Model file for the job. Use its own axes, mm. A direction names the side the tool comes from. Round coordinates to 2 decimals unless told otherwise and drop trailing zeros. Loops run counter-clockwise (first coordinate to the right, second up) from the corner with the lowest first, then second, coordinate; pieces in that order, holes last. Notation, with made-up numbers: (-32, 85.25) - (-22, 85.25) arc R14 ccw to (-22, 93.25) - close; hole circle Ø4 at (-33, 77). An arc over 180 degrees is marked (long way). Answer as a JSON object with one key per item and string values.
from build123d import *

# Parameters (mm, degrees)
BOX039_W                 = 5
BOX039_H                 = 12
BOX039_DEPTH             = 7.5
CYLINDER041_R            = 1.75
CYLINDER041_DEPTH        = 32
PRISM_DEPTH              = 10
SKETCH009_R              = 1
SKETCH009_W              = 24
SKETCH009_H              = 13
PAD004_DEPTH             = 30
CYLINDER039_R            = 1.75
CYLINDER039_DEPTH        = 32
CYLINDER039_ROLL_ANGLE   = -90
CYLINDER040_R            = 1.75
CYLINDER040_DEPTH        = 32
CYLINDER040_ROLL_ANGLE   = -90
BOX026_W                 = 19
BOX026_H                 = 15
BOX026_DEPTH             = 56
CHAMFER005_SIZE          = 3
FILLET054_R              = 0.5
CLONE013_PLACEMENT_ANGLE = -90


with BuildPart() as cubo015:
    # Box039 → Box039 (new body)
    with BuildSketch(Plane(origin=(9, 97, 127), x_dir=(1, 0, 0), z_dir=(0, 0, 1))):
        with Locations((2.5, 6)):
            Rectangle(BOX039_W, BOX039_H)
    extrude(amount=BOX039_DEPTH)


with BuildPart() as cilindro016:
    # Cylinder041 → Cylinder041 (new body)
    with BuildSketch(Plane(origin=(-5, 104, 125.85), x_dir=(0, -1, 0), z_dir=(1, 0, 0))):
        Circle(CYLINDER041_R)
    extrude(amount=CYLINDER041_DEPTH)


with BuildPart() as fusion030:
    # Prism → Prism (new body)
    with BuildSketch(Plane(origin=(6, 104, 125.85), x_dir=(0, -1, 0), z_dir=(1, 0, 0))):
        Polygon((3.3, 0), (1.65, 2.857884), (-1.65, 2.857884), (-3.3, 0), (-1.65, -2.857884), (1.65, -2.857884), align=None)
    extrude(amount=PRISM_DEPTH)

    # Fusion030: union Cilindro016
    add(cilindro016.part)


with BuildPart() as pad004:
    # Sketch009 → Pad004 (new body)
    with BuildSketch(Plane(origin=(38, -16, 143.25), x_dir=(0, 0, -1), z_dir=(1, 0, 0))):
        with Locations((37, 120)):
            Circle(SKETCH009_R)
        with Locations((9.5, 120)):
            Circle(SKETCH009_R)
        with Locations((23.25, 120)):
            Rectangle(SKETCH009_W, SKETCH009_H)
    extrude(amount=-PAD004_DEPTH)


with BuildPart() as cilindro014:
    # Cylinder039 → Cylinder039 (new body)
    with BuildSketch(Plane.XY):
        Circle(CYLINDER039_R)
    extrude(amount=CYLINDER039_DEPTH)


with BuildPart() as cilindro014_1:
    # Cylinder039 roll: moved
    add(cilindro014.part.rotate(Axis((0, 0, 0), (1, 0, 0)), CYLINDER039_ROLL_ANGLE))


with BuildPart() as cilindro014_2:
    # Cylinder039 placement: moved
    add(cilindro014_1.part.moved(Location((8, 90, 84))))


with BuildPart() as fusion029:
    # Cylinder040 → Cylinder040 (new body)
    with BuildSketch(Plane.XY):
        Circle(CYLINDER040_R)
    extrude(amount=CYLINDER040_DEPTH)


with BuildPart() as fusion029_1:
    # Cylinder040 roll: moved
    add(fusion029.part.rotate(Axis((0, 0, 0), (1, 0, 0)), CYLINDER040_ROLL_ANGLE))


with BuildPart() as fusion029_2:
    # Cylinder040 placement: moved
    add(fusion029_1.part.moved(Location((18, 90, 84))))

    # Fusion029: union Cilindro014
    add(cilindro014_2.part)


with BuildPart() as clone_of_arm:
    # Box026 → Box026 (new body)
    with BuildSketch(Plane(origin=(4, 98, 80), x_dir=(1, 0, 0), z_dir=(0, 0, 1))):
        with Locations((9.5, 7.5)):
            Rectangle(BOX026_W, BOX026_H)
    extrude(amount=BOX026_DEPTH)

    # Cut042: cut Fusion029
    add(fusion029_2.part, mode=Mode.SUBTRACT)

    # Cut043: cut Pad004
    add(pad004.part, mode=Mode.SUBTRACT)

    # Chamfer005
    chamfer005_edges = [clone_of_arm.edges().sort_by_distance(p)[0] for p in [
        (4, 105.5, 136),
        (13.5, 113, 136),
    ]]
    chamfer(chamfer005_edges, length=CHAMFER005_SIZE)

    # Cut044: cut Fusion030
    add(fusion030.part, mode=Mode.SUBTRACT)

    # Cut055: cut Cubo015
    add(cubo015.part, mode=Mode.SUBTRACT)

    # Fillet054
    fillet054_edges = [clone_of_arm.edges().sort_by_distance(p)[0] for p in [
        (11.5, 109, 134.5),
    ]]
    fillet(fillet054_edges, radius=FILLET054_R)


with BuildPart() as clone_of_arm_1:
    # Clone013 placement: moved
    add(clone_of_arm.part.moved(Location((-275, 70, 2.5))).rotate(Axis((-275, 70, 2.5), (0, 0, 1)), CLONE013_PLACEMENT_ANGLE))


with BuildPart() as clone_of_arm001:
    # Part__Mirroring008: instance of Clone of arm
    add(clone_of_arm_1.part.mirror(Plane(origin=(0, 0, 0), x_dir=(0, -1, 0), z_dir=(1, 0, 0))))


with BuildPart() as clone_of_arm001_1:
    # Part__Mirroring008 placement: moved
    add(clone_of_arm001.part.moved(Location((-478, 0, 0))))


solid = clone_of_arm001_1.part
1) Probe probe 1 along Y at (x, z) = (-310, 86.5); probe 2 along X at (y, z) = (65.2, 128.35); probe 3 along Z at (x, y) = (-303, 57.75). List the from-to ranges inside material, lowest first.
Values follow:
{"probe 1": "47 to 50.25, 53.75 to 60.25, 63.75 to 66", "probe 2": "-316 to -308.75, -305.25 to -301", "probe 3": "82.5 to 110.5, 137 to 138.5"}
2) Two-plate mould, pull along Z, no slides. Class faces 1 (the flat face through (-308, 66, 109)), 2 (the flat face through (-306, 64, 130)), 3 (the flat face through (-308.4, 64.5, 137)), 4 (the flat face through (-309, 57, 82.5)): pulls with the +Z half, pulls with the -Z half, needs draft (parallel to the pull), parting line crosses it, or undercut.
Values follow:
{"face 1": "needs draft", "face 2": "undercut", "face 3": "pulls with the +Z half", "face 4": "pulls with the -Z half"}
3) Slice it at D-D on x = -312.5. List the corners of the cut face in (y, z).
Values follow:
{"outline": "(47, 82.5) - (66, 82.5) - (66, 135.5) - (63, 138.5) - (47, 138.5) - (47, 134.5) - (62, 134.5) - (62, 110.5) - (47, 110.5) - close; hole circle Ø3.5 at (52, 86.5); hole circle Ø3.5 at (62, 86.5)"}
4) Tool access for faces 5 (the flat face through (-312, 59, 135)), 6 (the flat face through (-309.463, 63.014, 126.901)), 7 (the flat face through (-313.5, 54, 123)): list every direction of +Z, -Z, +X, -X, +Y, -Y with a clear straight run to the whole face (end or side of a thin tool).
Values follow:
{"face 5": "+X", "face 6": "-Y", "face 7": "+X, -Y"}
5) Slice it at B-B on z = 86.5. List the corners of the cut face in (x, y).
Values follow:
{"outline": "(-316, 47) - (-301, 47) - (-301, 50.25) - (-316, 50.25) - close; (-316, 53.75) - (-301, 53.75) - (-301, 60.25) - (-316, 60.25) - close; (-316, 63.75) - (-301, 63.75) - (-301, 66) - (-316, 66) - close"}
6) Drop flat-ended pins along their axis: P1, Ø1.2, axis at x = -307, z = 136.25, coming from the -Y side; P2, Ø1.5, axis at y = 59.5, z = 112.5, coming from the +X side; P3, Ø0.6, axis at y = 57.5, z = 135.5, coming from the +X side. Give the stop position or say it passes through.
Values follow:
{"P1": "y = 62", "P2": "x = -313.5", "P3": "x = -312"}
7) Slice it at A-A on x = -307. Count the separate pieces of the cut face and the enclosed holes in it, then the cut area to 3 significant figures.
Values follow:
{"separate pieces": "3", "enclosed holes": "2", "area": "598 mm²"}
8) Slice it at C-C on y = 52. List the corners of the cut face in (x, z).
Values follow:
{"outline": "(-316, 82.5) - (-301, 82.5) - (-301, 84.75) - (-316, 84.75) - close; (-316, 88.25) - (-301, 88.25) - (-301, 110.5) - (-313.5, 110.5) - (-313.5, 134.5) - (-301, 134.5) - (-301, 138.5) - (-313, 138.5) - (-316, 135.5) - close; hole circle Ø2 at (-307, 108.75); hole circle Ø2 at (-307, 136.25)"}
